Could you check a few things on this drawing? It's one solid part, dimensions in mm from its lowest x, y, z. A direction names the side the tool comes from. Round coordinates to 2 decimals unless told otherwise and drop trailing zeros. Order: outer loops, then holes, each group sorted by start corner. A loop starts at its lowest first (then second) coordinate and runs counter-clockwise, first axis right, second up. Notation, with made-up numbers: (75.5, 74.25) - (119.5, 74.25) arc R21 ccw to (119.5, 96.25) - close; hole circle Ø6 at (-9.75, -11.75). An arc over 180 degrees is marked (long way). Use one line per item in the form item = value.
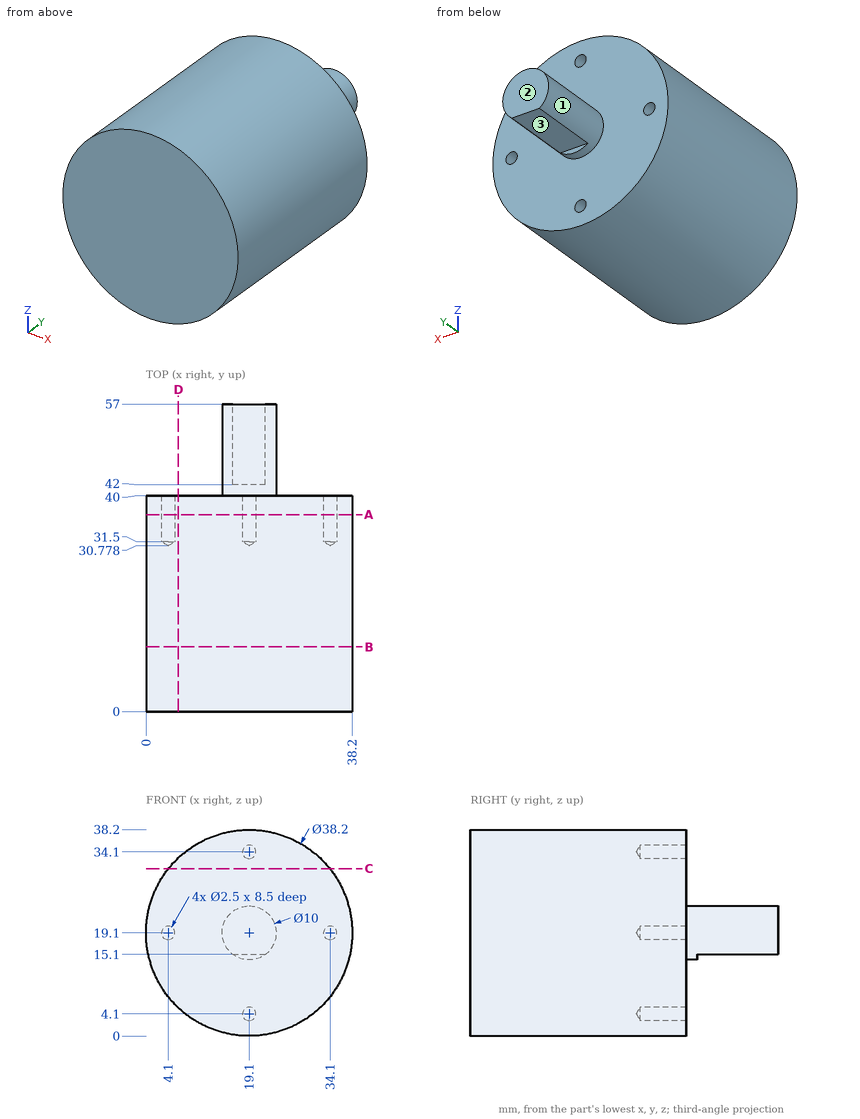
Item 1: For the marked faces 1, 2 and 3, which set-ups out of +Z, -Z, +X, -X, +Y, -Y let a thin tool reach every point of the face, with its end or its side?
Found:
face_1 = +Y
face_2 = +Z, -Z, +X, -X, +Y
face_3 = -Z, +X, -X, +Y
Item 2: Imagine slicing it at C-C on z = 31. Please give me the cut outline in (x, y), plus the area to 3 significant figures.
Found:
outline = (4.16, 0) - (34.04, 0) - (34.04, 40) - (4.16, 40) - close
area = 1,200 mm2
Item 3: I need wall thicknesses on L1, parallel to X at y = 35, z = 19; L2, parallel to Y at x = 4, z = 27.5; L3, parallel to X at y = 12, z = 19.5. Which ranges of each line are inside material? Lowest first, please.
Found:
L1 = 0 to 2.85, 5.35 to 32.85, 35.35 to 38.2
L2 = 0 to 40
L3 = 0 to 38.2
Item 4: Imagine slicing it at A-A on y = 36.5. Please give me the cut outline in (x, z).
Found:
outline = circle Ø38.2 at (19.1, 19.1); hole circle Ø2.5 at (4.1, 19.1); hole circle Ø2.5 at (19.1, 4.1); hole circle Ø2.5 at (19.1, 34.1); hole circle Ø2.5 at (34.1, 19.1)
Item 5: Imagine slicing it at B-B on y = 12. Please give me the cut outline in (x, z).
Found:
outline = circle Ø38.2 at (19.1, 19.1)
Item 6: Will these pins go through, and if not, where does the flat tip stop? P1, Ø1, axis at x = 4, z = 16, coming from the +Y side; P2, Ø1, axis at x = 16.5, z = 13, coming from the -Y side; P3, Ø1.8, axis at x = 19.5, y = 50, coming from the -Z side; P4, Ø4, axis at y = 10.5, z = 6.5, coming from the +X side.
Found:
P1 = 40
P2 = 0
P3 = 15.1
P4 = 34.99
Item 7: Imagine slicing it at D-D on x = 6. Please give me the cut outline in (y, z).
Found:
outline = (0, 5.2) - (40, 5.2) - (40, 33) - (0, 33) - close
